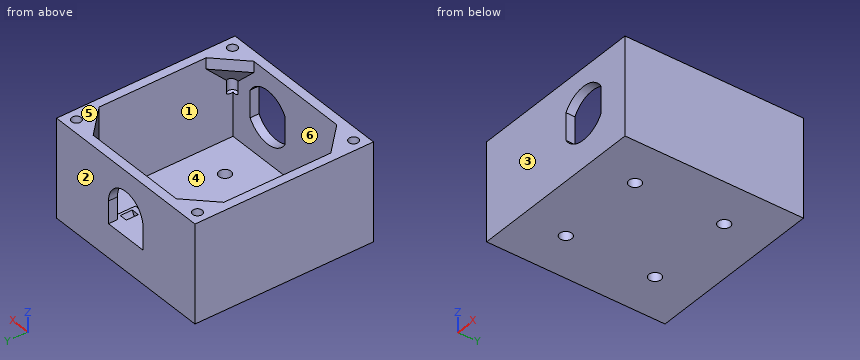
from build123d import *

# Parameters (mm, degrees)
SKETCH1_W                 = 50.8
SKETCH1_H                 = 50.8
BOSS_EXTRUDE1_DEPTH       = 2.54
SKETCH2_W                 = 50.8
SKETCH2_H                 = 50.8
SKETCH2_W_2               = 45.72
SKETCH2_H_2               = 45.72
BOSS_EXTRUDE2_DEPTH       = 25.4
CUT_EXTRUDE1_REACH        = 79.084
CUT_EXTRUDE3_REACH        = 79.084
BOSS_EXTRUDE3_DEPTH       = 25.4
CUT_EXTRUDE4_START        = -2.54
SKETCH8_W                 = 22.225
SKETCH8_H                 = 7.62
CUT_EXTRUDE4_DEPTH        = 12.7
LOFT1_START               = 36.295124673
LOFT1_DEPTH               = 4.399409051
F_6_32_TAPPED_HOLE1_D     = 2.7051
F_6_32_TAPPED_HOLE1_DEPTH = 12.7
F_6_32_TAPPED_HOLE1_TIP   = 0.81269403
F_6_CLEARANCE_HOLE1_D     = 3.429
SKETCH15_W                = 15.875
SKETCH15_H                = 6.35
BOSS_EXTRUDE5_DEPTH       = 6.985
CUT_EXTRUDE5_START        = -3.175
SKETCH16_R                = 7.62
SKETCH16_R_2              = 5.588
CUT_EXTRUDE5_DEPTH        = 1.7145


with BuildPart() as part:
    # Sketch1 → Boss-Extrude1 (new body)
    with BuildSketch(Plane.XY):
        with Locations((25.4, 25.4)):
            Rectangle(SKETCH1_W, SKETCH1_H)
    extrude(amount=BOSS_EXTRUDE1_DEPTH)

    # Sketch2 → Boss-Extrude2 (add)
    with BuildSketch(Plane.XY.offset(2.54)):
        with Locations((25.4, 25.4)):
            Rectangle(SKETCH2_W, SKETCH2_H)
        with Locations((25.4, 25.4)):
            Rectangle(SKETCH2_W_2, SKETCH2_H_2, mode=Mode.SUBTRACT)
    extrude(amount=BOSS_EXTRUDE2_DEPTH)

    # Sketch3 → Cut-Extrude1 (cut, up to next)
    with BuildSketch(Plane.XZ, mode=Mode.PRIVATE) as cut_extrude1_sk1:
        with BuildLine():
            Line((29.1465, 19.114540844), (29.1465, 11.365459156))
            ThreePointArc((29.1465, 11.365459156), (35.56, 7.747), (41.9735, 11.365459156))
            Line((41.9735, 11.365459156), (41.9735, 19.114540844))
            ThreePointArc((41.9735, 19.114540844), (35.56, 22.733), (29.1465, 19.114540844))
        make_face()
    cut_extrude1_tool1 = extrude(cut_extrude1_sk1.sketch, amount=-CUT_EXTRUDE1_REACH, mode=Mode.PRIVATE) & part.part
    add(cut_extrude1_tool1.solids().sort_by_distance((35.56, 0, 15.24))[0], mode=Mode.SUBTRACT)

    # Sketch4 → Cut-Extrude3 (cut, up to next)
    with BuildSketch(Plane(origin=(0, 50.8, 0), x_dir=(1, 0, 0), z_dir=(0, 1, 0)), mode=Mode.PRIVATE) as cut_extrude3_sk1:
        with BuildLine():
            Line((31.75, -15.875), (31.75, -9.525))
            Line((31.75, -9.525), (19.05, -9.525))
            Line((19.05, -9.525), (19.05, -15.875))
            ThreePointArc((19.05, -15.875), (25.4, -22.225), (31.75, -15.875))
        make_face()
    cut_extrude3_tool1 = extrude(cut_extrude3_sk1.sketch, amount=-CUT_EXTRUDE3_REACH, mode=Mode.PRIVATE) & part.part
    add(cut_extrude3_tool1.solids().sort_by_distance((25.4, 50.8, 15.282228))[0], mode=Mode.SUBTRACT)

    # Sketch6 → Boss-Extrude3 (add)
    with BuildSketch(Plane.XY.offset(2.54)):
        Polygon((2.54, 48.26), (10.16, 48.26), (2.54, 40.64), align=None)
        Polygon((48.26, 48.26), (48.26, 40.64), (40.64, 48.26), align=None)
        Polygon((48.26, 2.54), (48.26, 10.16), (40.64, 2.54), align=None)
        Polygon((2.54, 2.54), (2.54, 10.16), (10.16, 2.54), align=None)
    extrude(amount=BOSS_EXTRUDE3_DEPTH)

    # Sketch8 → Cut-Extrude4 (cut)
    with BuildSketch(Plane(origin=(50.8, 0, 0), x_dir=(0, 0, -1), z_dir=(1, 0, 0)).offset(CUT_EXTRUDE4_START)):
        with Locations((-13.6525, 6.35)):
            Rectangle(SKETCH8_W, SKETCH8_H)
    extrude(amount=-CUT_EXTRUDE4_DEPTH, mode=Mode.SUBTRACT)

    # Loft1: read off the stored shape, not the designer's step
    # Loft1 outline → Loft1 (add)
    with BuildSketch(Plane(origin=(0, 0, 0), x_dir=(0.8164965809277258, 0.40824829046386313, -0.40824829046386313), z_dir=(0.5773502691896258, -0.5773502691896258, 0.5773502691896258)).offset(LOFT1_START)):
        Polygon((33.441658713, 24.695704333), (24.109102793, 19.30755066), (33.441658713, 13.919396988), align=None)
    extrude(amount=LOFT1_DEPTH)

    # #6-32 Tapped Hole1
    with Locations(Plane.XY.offset(27.94)):
        with Locations((47.625, 3.175), (47.625, 47.625), (3.175, 47.625), (3.175, 3.175)):
            Hole(F_6_32_TAPPED_HOLE1_D / 2, depth=F_6_32_TAPPED_HOLE1_DEPTH)
            with Locations((0, 0, -(F_6_32_TAPPED_HOLE1_DEPTH + F_6_32_TAPPED_HOLE1_TIP / 2))):  # 118° drill point
                Cone(0, F_6_32_TAPPED_HOLE1_D / 2, F_6_32_TAPPED_HOLE1_TIP, mode=Mode.SUBTRACT)

    # #6 Clearance Hole1 (through all)
    with Locations(Plane.XY.offset(2.54)):
        with Locations((12.7, 38.1), (38.1, 38.1), (38.1, 12.7), (12.7, 12.7)):
            Hole(F_6_CLEARANCE_HOLE1_D / 2)

    # Sketch15 → Boss-Extrude5 (add)
    with BuildSketch(Plane.XY.offset(2.54)):
        with Locations((25.4, 45.085)):
            Rectangle(SKETCH15_W, SKETCH15_H)
    extrude(amount=BOSS_EXTRUDE5_DEPTH)

    # Sketch16 → Cut-Extrude5 (cut, symmetric)
    with BuildSketch(Plane.XZ.offset(-41.91).offset(CUT_EXTRUDE5_START)):
        with Locations((25.4, 12.065)):
            Circle(SKETCH16_R)
        with Locations((25.4, 12.065)):
            Circle(SKETCH16_R_2, mode=Mode.SUBTRACT)
    extrude(amount=CUT_EXTRUDE5_DEPTH, both=True, mode=Mode.SUBTRACT)


solid = part.part
Work out the finished part from the listing and answer in its coordinate system (mm). Face numbers are marked on the shaded views. A direction names the side the tool comes from. Round coordinates to 2 decimals unless told otherwise and drop trailing zeros. Loops run counter-clockwise (first coordinate to the right, second up) from the corner with the lowest first, then second, coordinate; pieces in that order, holes last. Notation, with made-up numbers: (-30, 87.25) -> (-16, 87.25) arc R14 cw to (-16, 99.25) -> close; hole circle Ø8 at (78, 71.5). An arc over 180 degrees is marked (long way). Use one line per item in the form item = value.
(1) Find section C-C on z = 12.25. Give the vertices of the cut face in (x, y), then the cut area to 3 significant figures.
Answer list:
outline = (0, 0) -> (29.15, 0) -> (29.15, 2.54) -> (10.16, 2.54) -> (2.54, 10.16) -> (2.54, 40.64) -> (10.16, 48.26) -> (19.05, 48.26) -> (19.05, 50.8) -> (0, 50.8) -> close; (31.75, 48.26) -> (40.64, 48.26) -> (48.26, 40.64) -> (48.26, 2.54) -> (41.97, 2.54) -> (41.97, 0) -> (50.8, 0) -> (50.8, 50.8) -> (31.75, 50.8) -> close
area = 513 mm2
(2) For a pull along Y with two mould halves and no side action, classify the marked faces 3, 4, 5 and 6 as released by +Y, released by -Y, zero draft, split by the parting line, or undercut.
Answer list:
face_3 = released by -Y
face_4 = undercut
face_5 = zero draft
face_6 = undercut
(3) Find section A-A on x = 25.4. Give the vertices of the cut face in (y, z) (1 decimal).
Answer list:
outline = (0, 0) -> (50.8, 0) -> (50.8, 9.5) -> (41.9, 9.5) -> (41.9, 2.5) -> (2.5, 2.5) -> (2.5, 27.9) -> (0, 27.9) -> close; (48.3, 22.2) -> (50.8, 22.2) -> (50.8, 27.9) -> (48.3, 27.9) -> close; hole (43.4, 4.4) -> (46.8, 4.4) -> (46.8, 6.5) -> (43.4, 6.5) -> close
(4) Straight lines are drawn through the part: line 1 (Y direction, x = 12.7, z = 0.75); line 2 (X direction, y = 25, z = 24.5); line 3 (X direction, y = 47.5, z = 25). For each, find the intervals that lie inside material, in ascending order.
Answer list:
line_1 = 0 to 10.99, 14.41 to 36.39, 39.81 to 50.8
line_2 = 0 to 2.54, 48.26 to 50.8
line_3 = 0 to 1.83, 4.52 to 9.4, 41.4 to 46.28, 48.97 to 50.8
(5) Flat-ended cylindrical pins translate along their axes: P1, Ø1, axis at x = 24, y = 21, coming from the +Z side; P2, Ø4, axis at x = 30.5, y = 39, coming from the -Z side; P3, Ø4.5, axis at x = 23.5, y = 45.5, coming from the +Z side (3 decimals); P4, Ø1, axis at x = 38, z = 14, coming from the -Y side. Find the tip coordinate at first contact, or state that the pin passes through.
Answer list:
P1 = 2.54
P2 = 0
P3 = 9.525
P4 = 48.26
(6) Find section B-B on y = 38.1. Give the vertices of the cut face in (x, z).
Answer list:
outline = (0, 0) -> (10.99, 0) -> (10.99, 2.54) -> (2.54, 2.54) -> (2.54, 27.94) -> (0, 27.94) -> close; (14.41, 0) -> (36.39, 0) -> (36.39, 2.54) -> (14.41, 2.54) -> close; (39.81, 0) -> (50.8, 0) -> (50.8, 27.94) -> (48.26, 27.94) -> (48.26, 2.54) -> (39.81, 2.54) -> close
(7) A tool of negligible diameter and unlimited length cuts with its end or side. For the marked faces 1 and 2, from which of +Z, -Z, +X, -X, +Y, -Y can it reach the whole face along a straight path? Write none if from no direction.
Answer list:
face_1 = none
face_2 = +Z, -Z, +X, -X, +Y
